Input: part model. Units: mm. Frame: model coordinates. A direction names the side the tool comes from. Coordinates: 2 decimals unless noted, no trailing zeros. Order: outer loops, then holes, each group sorted by start corner. A loop starts at its lowest first (then second) coordinate and runs counter-clockwise, first axis right, second up. Notation, with made-up numbers: M 60.5,-5.75 L 93.5,-5.75 A23 ccw 93.5,22.25 Z; hole C 52.25,70.25 d1. An arc over 180 degrees is marked long. Answer in a Markdown table with one row per item.
from build123d import *

# Parameters (mm, degrees)
SKETCH4_W           = 24.633837396
SKETCH4_H           = 19.082768461
SKETCH4_W_2         = 5
SKETCH4_H_2         = 5
MAINBRACKET_DEPTH   = 3.5
SKETCH3_R           = 2
BOSS_EXTRUDE2_DEPTH = 13
SKETCH6_R           = 1.5
BOSS_EXTRUDE3_DEPTH = 5


with BuildPart() as part:
    # Sketch4 → MainBracket (new body)
    with BuildSketch(Plane(origin=(0, 0, 0), x_dir=(1, 0, 0), z_dir=(0, 1, 0))):
        Polygon((-25.001052975, 23.597895529), (25.52718448, 23.597895529), (27.52718448, 21.597895529), (27.52718448, 18.397895529), (25.52718448, 16.397895529), (15.338231538, 16.397895529), (15.338231538, -31.590979949), (12.338231538, -34.590979949), (-1.661768462, -34.590979949), (-4.661768462, -31.590979949), (-4.661768462, -15.921260677), (-16.583029139, -4), (-16.583029139, 16.421906692), (-25.001052975, 16.421906692), (-27.001052975, 18.421906692), (-27.001052975, 21.597895529), align=None)
        with Locations((0.008956485, 13.000441896)):
            Rectangle(SKETCH4_W, SKETCH4_H, mode=Mode.SUBTRACT)
        with Locations((-0.204070078, -11.047717724)):
            Rectangle(SKETCH4_W_2, SKETCH4_H_2, mode=Mode.SUBTRACT)
    extrude(amount=MAINBRACKET_DEPTH)

    # Sketch3 → Boss-Extrude2 (add)
    with BuildSketch(Plane(origin=(0, 0, 0), x_dir=(1, 0, 0), z_dir=(0, 1, 0))):
        with Locations(Location((-24.011269627, 19.663273311, 0), (0, 0, 270))):
            Circle(SKETCH3_R)
        with Locations(Location((24.107482847, 18.27469294, 0), (0, 0, 270))):
            Circle(SKETCH3_R)
        with Locations(Location((8.917908931, -32.088026328, 0), (0, 0, 270))):
            Circle(SKETCH3_R)
    extrude(amount=-BOSS_EXTRUDE2_DEPTH)

    # Sketch6 → Boss-Extrude3 (add)
    with BuildSketch(Plane.XZ.offset(13)):
        with Locations(Location((-24.011269627, -19.663273311, 0), (0, 0, 270))):
            Circle(SKETCH6_R)
        with Locations(Location((8.917908931, 32.088026328, 0), (0, 0, 270))):
            Circle(SKETCH6_R)
        with Locations(Location((24.107482847, -18.27469294, 0), (0, 0, 270))):
            Circle(SKETCH6_R)
    extrude(amount=BOSS_EXTRUDE3_DEPTH)


solid = part.part
1) Contact query for flat-ended pins moving along their axis: pin 1 (4 mm diameter, centred on x = -12, y = -1, fed in from +Z); pin 2 (4 mm diameter, centred on y = 2.5, z = 11.5, fed in from -X); pin 3 (1 mm diameter, centred on y = 1, z = 19.5, fed in from +X). Output: stop coordinate, or through.
Resolved:
| item | result |
|---|---|
| pin 1 | stops at z = 10.32 |
| pin 2 | stops at x = -11.08 |
| pin 3 | stops at x = 15.34 |
2) Cut plane D-D, the plane y = -14.5. Output: boundary loops of the cut face in (x, z), and give its area (3 significant figures).
Resolved:
| item | result |
|---|---|
| outline | C -24.01,-19.66 d3; C 8.92,32.09 d3; C 24.11,-18.27 d3 |
| area | 21.2 mm2 |
3) Reachability of faces 1 (the face through (-21, 2, -16.422)), 2 (the face through (2, 3.5, 3)), 3 (the face through (0, 2, -22.542)), 4 (the face through (8.01, -15.46, 33.28)) from +Z, -Z, +X, -X, +Y, -Y: full face, straight path, thin tool, end or side. Return the list, or none.
Resolved:
| item | result |
|---|---|
| face 1 | +Z, -X, +Y, -Y |
| face 2 | +Z, -Z, +X, -X, +Y |
| face 3 | +Y, -Y |
| face 4 | -Y |
4) Material intervals for probe 1 along Y at (x, z) = (4, -1); probe 2 along Z at (x, y) = (18, 0.25); probe 3 along Z at (x, y) = (9.5, -14), sorted ascending.
Resolved:
| item | result |
|---|---|
| probe 1 | y = 0 to 3.5 |
| probe 2 | z = -23.6 to -16.4 |
| probe 3 | z = 30.71 to 33.47 |
5) Cut plane A-A, the plane z = -13.5. Output: boundary loops of the cut face in (x, y).
Resolved:
| item | result |
|---|---|
| outline | M -16.58,0 L -12.31,0 L -12.31,3.5 L -16.58,3.5 Z; M 12.33,0 L 15.34,0 L 15.34,3.5 L 12.33,3.5 Z |
6) Cut plane C-C, the plane x = -10. Output: boundary loops of the cut face in (y, z), and give its area (3 significant figures).
Resolved:
| item | result |
|---|---|
| outline | M 0,-23.6 L 3.5,-23.6 L 3.5,-22.54 L 0,-22.54 Z; M 0,-3.46 L 3.5,-3.46 L 3.5,10.58 L 0,10.58 Z |
| area | 52.8 mm2 |
7) Mould query, pull axis X, two halves, no side actions, for faces 5 (the face through (0, 2, -3.459)), 6 (the face through (21, 2, -16.398)), 7 (the face through (22.89, -6.41, -19.86)), 8 (the face through (-27.001, 2, -20)). Classes: +X half, -X half, draft (parallel to the pull), parting line (faces both ways), or undercut.
Resolved:
| item | result |
|---|---|
| face 5 | undercut |
| face 6 | draft |
| face 7 | undercut |
| face 8 | -X half |
8) Cut plane B-B, the plane x = -1. Output: boundary loops of the cut face in (y, z), and give its area (3 significant figures).
Resolved:
| item | result |
|---|---|
| outline | M 0,-23.6 L 3.5,-23.6 L 3.5,-22.54 L 0,-22.54 Z; M 0,-3.46 L 3.5,-3.46 L 3.5,8.55 L 0,8.55 Z; M 0,13.55 L 3.5,13.55 L 3.5,34.59 L 0,34.59 Z |
| area | 119 mm2 |
